Verification items for the finished model (mm, model axes). A direction names the side the tool comes from. Coordinates: 2 decimals unless noted, no trailing zeros. Write each loop counter-clockwise with the first axis right and the second up, starting at its lowest first coordinate (ties: lowest second). Pieces come first, ordered by that corner, then holes. Notation, with made-up numbers: (-8, 31) - (36, 31) arc R29 ccw to (36, 61) - close; hole circle Ø6 at (1, 64). An arc over 180 degrees is marked (long way). Use CSV: the item, a comma, the result in double quotes. Start each with the question number.
```python
from build123d import *

# Parameters (mm, degrees)
BOSS_EXTRUDE1_DEPTH                        = 304.8
CUT_EXTRUDE1_DEPTH                         = 307.860095361
CUT_EXTRUDE2_DEPTH                         = 307.860095361
CUT_EXTRUDE2_DEPTH_BACK                    = 307.860095361
SKETCH3_R                                  = 2.413
CUT_EXTRUDE3_DEPTH                         = 307.860095361
CUT_EXTRUDE3_DEPTH_BACK                    = 307.860095361
SKETCH4_R                                  = 2.413
CSK_FOR_10_FLAT_HEAD_MACHINE_SCREW_2_COUNT = 2
CSK_FOR_10_FLAT_HEAD_MACHINE_SCREW_2_PITCH = 19.05


with BuildPart() as part:
    # Sketch1 → Boss-Extrude1 (new body)
    with BuildSketch(Plane(origin=(0, 0, 0), x_dir=(1, 0, 0), z_dir=(0, 1, 0))):
        Polygon((-15.875, -15.875), (-12.7, -15.875), (-12.7, 12.7), (12.7, 12.7), (12.7, -15.875), (15.875, -15.875), (15.875, 15.875), (-15.875, 15.875), align=None)
    extrude(amount=BOSS_EXTRUDE1_DEPTH)

    # Sketch2 → Cut-Extrude1 (cut, through all)
    with BuildSketch(Plane(origin=(15.875, 0, 0), x_dir=(0, 0, -1), z_dir=(1, 0, 0))):
        Polygon((-15.875, 0), (15.875, 37.838176565), (15.875, 0), align=None)
    extrude(amount=-CUT_EXTRUDE1_DEPTH, mode=Mode.SUBTRACT)

    # Sketch3 → Cut-Extrude2 (cut, two sides: drawn at the far end of the back side and taken through both)
    with BuildSketch(Plane(origin=(15.875, 0, 0), x_dir=(0, 0, -1), z_dir=(1, 0, 0)).offset(-CUT_EXTRUDE2_DEPTH_BACK)):
        with Locations((-6.35, 273.05)):
            Circle(SKETCH3_R)
        with Locations((-6.35, 82.55)):
            Circle(SKETCH3_R)
        with Locations((-6.35, 146.05)):
            Circle(SKETCH3_R)
    extrude(amount=CUT_EXTRUDE2_DEPTH + CUT_EXTRUDE2_DEPTH_BACK, mode=Mode.SUBTRACT)

    # Sketch4 → Cut-Extrude3 (cut, two sides: drawn at the far end of the back side and taken through both)
    with BuildSketch(Plane(origin=(15.875, 0, 0), x_dir=(0, 0, -1), z_dir=(1, 0, 0)).offset(-CUT_EXTRUDE3_DEPTH_BACK)):
        with Locations((0, 48.274473485)):
            Circle(SKETCH4_R)
        with Locations((0, 38.114473485)):
            Circle(SKETCH4_R)
    extrude(amount=CUT_EXTRUDE3_DEPTH + CUT_EXTRUDE3_DEPTH_BACK, mode=Mode.SUBTRACT)

    # Sketch11 → CSK for #10 Flat Head Machine Screw (100)1 (revolve, cut)
    with BuildSketch(Plane(origin=(12.7, 219.033346522, -6.35), x_dir=(0, 0, 1), z_dir=(0, 1, 0))):
        Polygon((0, 0), (0, 3.175), (2.5527, 3.175), (2.5527, 1.960808018), (4.8895, 0), align=None)
    csk_for_10_flat_head_machine_screw_100 = revolve(axis=Axis((6.35, 219.033346522, -6.35), (1, 0, 0)), mode=Mode.SUBTRACT)

    # CSK for _10 Flat Head Machine Screw  2: CSK for #10 Flat Head Machine Screw (100)1 ×2
    with Locations(*[Vector(0, -0.766044443118978, 0.6427876096865395) * (i * CSK_FOR_10_FLAT_HEAD_MACHINE_SCREW_2_PITCH) for i in range(1, CSK_FOR_10_FLAT_HEAD_MACHINE_SCREW_2_COUNT)]):
        add(csk_for_10_flat_head_machine_screw_100, mode=Mode.SUBTRACT)

    # Mirror4: CSK for #10 Flat Head Machine Screw (100)1 across plane
    add(csk_for_10_flat_head_machine_screw_100.mirror(Plane(origin=(0, 0, 0), x_dir=(0, 0, 1), z_dir=(1, 0, 0))), mode=Mode.SUBTRACT)

    # Mirror4 copy 1 sketch → Mirror4 copy 1 (revolve, cut)
    with BuildSketch(Plane(origin=(-12.7, 204.440199881, 5.895103965), x_dir=(0, 0, 1), z_dir=(0, 1, 0))):
        Polygon((0, 0), (0, -3.175), (2.5527, -3.175), (2.5527, -1.960808018), (4.8895, 0), align=None)
    revolve(axis=Axis((-6.35, 204.440199881, 5.895103965), (1, 0, 0)), mode=Mode.SUBTRACT)


solid = part.part
```
Q1. Scan lines: line 1 along X through (y, z) = (243, -6) (3 decimals); line 2 along Z through (x, y) = (-14.45, 273.05) (3 decimals); line 3 along Y through (x, z) = (13.6, 6.35). Record each from-to range of solid material in increasing order. Write a range as from..to.
Q2. Tool access check on faces 1 (the flat face through (12.7, 150, 1)), 2 (the conical face through (14.54, 207.07, 5.31)), 3 (the cylindrical face through (-14.31, 35.76, 0.52)). Record the directions out of +Z, -Z, +X, -X, +Y, -Y that give a thin tool (end or side, any length) a straight path to the whole face; none if there is none.
Q3. Gauge pin test, flat ends, axial feed: pin 1 (4 mm diameter, centred on y = 38.11, z = 0, fed in from -X); pin 2 (5 mm diameter, centred on x = -1.5, y = 35, fed in from +Z); pin 3 (3 mm diameter, centred on x = 11.5, z = -5, fed in from -Y). Record the tip position at first contact, or that the pin passes through.
Q4. Cross-section at A-A (z = -6.35). Record the cut outline in (x, y) (3 decimals).
Q5. Release check for a two-part mould opening along Z. For faces 4 (the flat face through (0, 168, -12.7)), 5 (the cylindrical face through (14.265, 50.667, 0.314)), 6 (the cylindrical face through (15.259, 216.502, -6.682)), 7 (the flat face through (-12.7, 150, 2)) record: released by +Z, released by -Z, zero draft, split by the parting line, or undercut.
Q6. Cross-section at C-C (x = -7.5). Record the cut outline in (y, z) (3 decimals).
Q7. Cross-section at B-B (y = 257). Record the cut outline in (x, z) (3 decimals).
Reply:
1,line 1,"-15.875..-12.7, 12.7..15.875"
1,line 2,"-15.875..3.937, 8.763..15.875"
1,line 3,"11.35..80.14, 84.96..143.64, 148.46..200.65, 208.23..270.64, 275.46..304.8"
2,face 1,"+Z, +Y, -Y"
2,face 2,"none"
2,face 3,"+X, -X"
3,pin 1,"through"
3,pin 2,"z = -12.7"
3,pin 3,"y = 23.81"
4,outline,"(-15.875, 26.487) - (-12.7, 26.487) - (-12.7, 214.144) - (-14.661, 216.481) - (-15.875, 216.481) - close; (-15.875, 221.586) - (-14.661, 221.586) - (-12.7, 223.923) - (-12.7, 304.8) - (-15.875, 304.8) - close; (12.7, 26.487) - (15.875, 26.487) - (15.875, 216.481) - (14.661, 216.481) - (12.7, 214.144) - close; (12.7, 223.923) - (14.661, 221.586) - (15.875, 221.586) - (15.875, 304.8) - (12.7, 304.8) - close"
5,face 4,"released by +Z"
5,face 5,"undercut"
5,face 6,"undercut"
5,face 7,"zero draft"
6,outline,"(34.054, -12.7) - (37.838, -15.875) - (304.8, -15.875) - (304.8, -12.7) - close"
7,outline,"(-15.875, -15.875) - (15.875, -15.875) - (15.875, 15.875) - (12.7, 15.875) - (12.7, -12.7) - (-12.7, -12.7) - (-12.7, 15.875) - (-15.875, 15.875) - close"
